Geometry: final body of the model. Coordinates: model frame, mm. A direction names the side the tool comes from. Give positions to 0.01 mm unless a question says otherwise; leave off trailing zeros. Order: outer loops, then holes, each group sorted by start corner. A loop starts at its lowest first (then second) coordinate and runs counter-clockwise, first axis right, second up. Notation, with made-up numbers: (-14.75, 72) - (-7.75, 72) arc R28 cw to (-7.75, 105) - close; hole circle Ø11 at (59, 68). An arc over 180 degrees is marked (long way). Use one line per item in the form item = value.
from build123d import *

# Parameters (mm, degrees)
F1_DEPTH = 63.5
F2_DEPTH = 12.7
F3_DEPTH = 7.9375
F5_R     = 5.08


with BuildPart() as f1:
    # F0 (on Front) → F1 (new body, symmetric)
    with BuildSketch(Plane.XZ):
        Polygon((41.275, -9.525), (41.275, 9.525), (22.225, 9.525), (-41.275, 9.525), (-41.275, -9.525), align=None)
    extrude(amount=F1_DEPTH, both=True)

    # F0 (on Front) → F2 (join, symmetric)
    with BuildSketch(Plane.XZ):
        with BuildLine():
            Line((22.225, 9.525), (41.275, 9.525))
            Line((41.275, 9.525), (41.275, 27.0002))
            ThreePointArc((41.275, 27.0002), (45.9246798487, 38.2255201513), (57.15, 42.8752))
            Line((57.15, 42.8752), (57.2056991218, 42.8752))
            Line((57.2056991218, 42.8752), (57.2056991218, 61.9252))
            Line((57.2056991218, 61.9252), (57.15, 61.9252))
            add(Edge.make_bspline(
                [(57.15, 61.9252), (56.1205296963, 61.8926068548), (55.0840965314, 61.8462999184), (54.0416201499, 61.786599637)],
                knots=[0, 0, 0, 0, 2.6733285205, 2.6733285205, 2.6733285205, 2.6733285205], degree=3))
            ThreePointArc((54.0416201499, 61.786599637), (31.3787389592, 50.5713206642), (22.225, 27.0002))
            Line((22.225, 27.0002), (22.225, 9.525))
        make_face()
        Polygon((57.2056991218, 61.9252), (57.2056991218, 42.8752), (85.6222819207, 42.8752), (85.7045002339, 61.9252), align=None)
    extrude(amount=F2_DEPTH, both=True)

    # F0 (on Front) → F3 (join, symmetric)
    with BuildSketch(Plane.XZ):
        with BuildLine():
            Line((-41.275, 9.525), (22.225, 9.525))
            Line((22.225, 9.525), (22.225, 27.0002))
            ThreePointArc((22.225, 27.0002), (31.3787389592, 50.5713206642), (54.0416201499, 61.786599637))
            add(Edge.make_bspline(
                [(54.0416201499, 61.786599637), (11.6024052654, 59.3562011022), (-40.8522579656, 34.7289555266), (-41.275, 9.525)],
                knots=[2.6733285205, 2.6733285205, 2.6733285205, 2.6733285205, 111.5045361635, 111.5045361635, 111.5045361635, 111.5045361635], degree=3))
        make_face()
    extrude(amount=F3_DEPTH, both=True)

    # F0 (on Front) → F4 (revolve)
    with BuildSketch(Plane.XZ):
        Polygon((85.7045002339, 61.9252), (85.6222819207, 42.8752), (85.6016725302, 38.1), (108.0056991218, 38.1), (108.0056991218, 66.675), (85.725, 66.675), align=None)
    revolve(axis=Axis((85.6633362651, 0, 52.3875), (0.0043158818, 0, 0.9999906865)))

    # F5
    f5_edges = [f1.edges().sort_by_distance(p)[0] for p in [
        (-41.275, 63.5, 0),
        (-41.275, -63.5, 0),
        (41.275, -63.5, 0),
        (41.275, 63.5, 0),
    ]]
    fillet(f5_edges, radius=F5_R)


solid = f1.part
(1) Cut plane A-A on z = -1. Output: boundary loops of the cut face in (x, y) (3 decimals).
Computed values:
outline = (-41.275, -58.42) arc R5.08 ccw to (-36.195, -63.5) - (36.195, -63.5) arc R5.08 ccw to (41.275, -58.42) - (41.275, 58.42) arc R5.08 ccw to (36.195, 63.5) - (-36.195, 63.5) arc R5.08 ccw to (-41.275, 58.42) - close
(2) Reachability of faces 1 (the face through (22.225, 10, 18)), 2 (the face through (31.625, -10.352, 50.837)) from +Z, -Z, +X, -X, +Y, -Y: full face, straight path, thin tool, end or side. Return the list, or none.
Computed values:
face_1 = +Z, -X, +Y
face_2 = +Z, -X, -Y
(3) Ray query, line 1 along Y through (x, z) = (3, 14); line 2 along Z through (x, y) = (22.5, -36) (3 decimals); line 3 along Z through (x, y) = (56.5, -2). Return the intervals inside material, ascending.
Computed values:
line_1 = -7.94 to 7.94
line_2 = -9.525 to 9.525
line_3 = 42.86 to 61.9
(4) Contact query for flat-ended pins moving along their axis: pin 1 Ø5 at (y, z) = (11.5, 14.5) entering from -X (3 decimals); pin 2 Ø1.5 at (x, y) = (75, -9) entering from -Z; pin 3 Ø3 at (x, y) = (-7.5, -25) entering from +Z (3 decimals). Output: stop coordinate, or through.
Computed values:
pin_1 = 22.225
pin_2 = 38.2
pin_3 = 9.525
(5) Cut plane B-B on y = -48. Output: boundary loops of the cut face in (x, z) (3 decimals), plus the area to 3 significant figures.
Computed values:
outline = (-41.275, -9.525) - (41.275, -9.525) - (41.275, 9.525) - (-41.275, 9.525) - close
area = 1,570 mm²
(6) Pull-direction query (X, two-part tool) for faces 3 (the face through (1, 35, 9.525)), 4 (the face through (39.8, -62, 0.1)), 5 (the face through (61, 0, 42.875)); classes: released by +X, released by -X, zero draft, split by the parting line, or undercut.
Computed values:
face_3 = zero draft
face_4 = released by +X
face_5 = undercut
